```python
from build123d import *

# Parameters (mm, degrees)
SKETCH1_W                     = 100
SKETCH1_H                     = 400
BOSS_EXTRUDE1_DEPTH           = 3.175
M4_CLEARANCE_HOLE2_D          = 4.5
SKETCH7_W                     = 400
SKETCH7_H                     = 3.175
BOSS_EXTRUDE2_DEPTH           = 20
M4_CLEARANCE_HOLE1_D          = 4.5
SKETCH13_W                    = 17.5
SKETCH13_H                    = 265
SKETCH13_W_2                  = 58
SKETCH13_H_2                  = 69.5
SKETCH13_W_3                  = 4.5
SKETCH13_H_3                  = 66
SKETCH13_H_4                  = 10
SKETCH13_H_5                  = 29.5
SKETCH13_H_6                  = 75
CUT_EXTRUDE1_DEPTH            = 3.175
FILLET1_R                     = 10
SKETCH14_W                    = 120
SKETCH14_H                    = 250.5
CUT_EXTRUDE2_DEPTH            = 3.175
M4_CLEARANCE_HOLE3_AT_2_COUNT = 2
M4_CLEARANCE_HOLE3_AT_2_PITCH = 26.666666667


with BuildPart() as part:
    # Sketch1 → Boss-Extrude1 (new body)
    with BuildSketch(Plane(origin=(0, 0, 0), x_dir=(1, 0, 0), z_dir=(0, 1, 0))):
        Rectangle(SKETCH1_W, SKETCH1_H)
    extrude(amount=BOSS_EXTRUDE1_DEPTH)

    # M4 Clearance Hole2 (through all)
    with Locations(Plane(origin=(0, 3.175, 0), x_dir=(1, 0, 0), z_dir=(0, 1, 0))):
        with Locations((-40, 190), (40, 190), (40, -190), (-40, -190), (-40, 95), (40, 95)):
            Hole(M4_CLEARANCE_HOLE2_D / 2)

    # Sketch7 → Boss-Extrude2 (add)
    with BuildSketch(Plane(origin=(50, 0, 0), x_dir=(0, 0, -1), z_dir=(1, 0, 0))):
        with Locations((0, 1.5875)):
            Rectangle(SKETCH7_W, SKETCH7_H)
    extrude(amount=BOSS_EXTRUDE2_DEPTH)

    # M4 Clearance Hole1 (through all)
    with Locations(Plane(origin=(0, 3.175, 0), x_dir=(1, 0, 0), z_dir=(0, 1, 0))):
        with Locations((55.5, -140.5), (55.5, -110.5), (-22.5, -110.5), (-22.5, -140.5), (-22.5, -24.5), (-22.5, 5.5), (55.5, 5.5), (55.5, -24.5)):
            Hole(M4_CLEARANCE_HOLE1_D / 2)

    # Sketch13 → Cut-Extrude1 (cut)
    with BuildSketch(Plane(origin=(0, 3.175, 0), x_dir=(1, 0, 0), z_dir=(0, 1, 0))):
        with Locations((-41.25, -47.5)):
            Rectangle(SKETCH13_W, SKETCH13_H)
        with Locations((16.5, 50.25)):
            Rectangle(SKETCH13_W_2, SKETCH13_H_2)
        with Locations((67.75, -47.5)):
            Rectangle(SKETCH13_W_3, SKETCH13_H)
        with Locations((16.5, -67.5)):
            Rectangle(SKETCH13_W_2, SKETCH13_H_3)
        with Locations((16.5, -125.5)):
            Rectangle(SKETCH13_W_2, SKETCH13_H_4)
        with Locations((16.5, -165.25)):
            Rectangle(SKETCH13_W_2, SKETCH13_H_5)
        with Locations((-41.25, 142.5)):
            Rectangle(SKETCH13_W, SKETCH13_H_6)
        with Locations((16.5, 142.5)):
            Rectangle(SKETCH13_W_2, SKETCH13_H_6)
        with Locations((67.75, 142.5)):
            Rectangle(SKETCH13_W_3, SKETCH13_H_6)
        with Locations((16.5, -9.5)):
            Rectangle(SKETCH13_W_2, SKETCH13_H_4)
    extrude(amount=-CUT_EXTRUDE1_DEPTH, mode=Mode.SUBTRACT)

    # Fillet1
    # the kernel refuses this fillet: 10 mm, written as the material it takes off along each edge
    with BuildSketch(Plane(origin=(70, 24.054116361, -180), x_dir=(0, 0, -1), z_dir=(0, -1, 0)), Plane(origin=(70, 24.054116361, -85), x_dir=(0, 0, -1), z_dir=(0, -1, 0))) as fillet1_piece_1:
        with BuildLine():
            CenterArc((8.351646544, -10), FILLET1_R, 90, 56.632987031)
            Line((0, -4.5), (-0.167032931, -4.39))
            ThreePointArc((-0.167032931, -4.39), (-0.2, -2.25), (-0.2, 0))
            Line((-0.2, 0), (0, 0.2))
            Line((0, 0.2), (8.351646544, 0.2))
            Line((8.351646544, 0.2), (8.351646544, 0))
        make_face()
    extrude(amount=44.933232721, mode=Mode.SUBTRACT)
    with BuildSketch(Plane(origin=(70, -25, -200), x_dir=(-1, 0, 0), z_dir=(0, 1, 0)), Plane(origin=(-50, -25, -200), x_dir=(0, 0, 1), z_dir=(0, 1, 0)), Plane(origin=(70, 28.175, 200), x_dir=(-1, 0, 0), z_dir=(0, -1, 0)), Plane(origin=(-50, -25, 200), x_dir=(1, 0, 0), z_dir=(0, 1, 0))) as fillet1_piece_2:
        with BuildLine():
            CenterArc((FILLET1_R, FILLET1_R), FILLET1_R, 180, 90)
            Line((0, FILLET1_R), (-FILLET1_R * 0.02, FILLET1_R))
            Line((-FILLET1_R * 0.02, FILLET1_R), (-FILLET1_R * 0.02, -FILLET1_R * 0.02))
            Line((-FILLET1_R * 0.02, -FILLET1_R * 0.02), (FILLET1_R, -FILLET1_R * 0.02))
            Line((FILLET1_R, -FILLET1_R * 0.02), (FILLET1_R, 0))
        make_face()
    extrude(amount=53.175, mode=Mode.SUBTRACT)
    with BuildSketch(Plane(origin=(-50, 28.175, -180), x_dir=(1, 0, 0), z_dir=(0, -1, 0)), Plane(origin=(-50, 28.175, -85), x_dir=(1, 0, 0), z_dir=(0, -1, 0)), Plane(origin=(-50, 28.175, -105), x_dir=(0, 0, 1), z_dir=(0, -1, 0)), Plane(origin=(-50, 28.175, 180), x_dir=(0, 0, 1), z_dir=(0, -1, 0))) as fillet1_piece_3:
        with BuildLine():
            CenterArc((FILLET1_R, -FILLET1_R), FILLET1_R, 90, 90)
            Line((0, -FILLET1_R), (-FILLET1_R * 0.02, -FILLET1_R))
            Line((-FILLET1_R * 0.02, -FILLET1_R), (-FILLET1_R * 0.02, FILLET1_R * 0.02))
            Line((-FILLET1_R * 0.02, FILLET1_R * 0.02), (FILLET1_R, FILLET1_R * 0.02))
            Line((FILLET1_R, FILLET1_R * 0.02), (FILLET1_R, 0))
        make_face()
    extrude(amount=53.175, mode=Mode.SUBTRACT)
    with BuildSketch(Plane(origin=(70, 24.054116361, -105), x_dir=(-1.0, 0, 1.5347723092402606e-12), z_dir=(0, -1, 0))) as fillet1_piece_4:
        with BuildLine():
            CenterArc((10, -8.351646544), FILLET1_R, 123.367012969, 56.632987031)
            Line((0, -8.351646544), (-0.2, -8.351646544))
            Line((-0.2, -8.351646544), (-0.2, 0))
            Line((-0.2, 0), (0, 0.2))
            ThreePointArc((0, 0.2), (2.25, 0.2), (4.39, 0.167032931))
            Line((4.39, 0.167032931), (4.5, 0))
        make_face()
    extrude(amount=44.933232721, mode=Mode.SUBTRACT)
    with BuildSketch(Plane(origin=(70, 24.054116361, 180), x_dir=(0, 0, 1), z_dir=(0, -1, 0))) as fillet1_piece_5:
        with BuildLine():
            CenterArc((8.351646544, 10), FILLET1_R, 213.367012969, 56.632987031)
            Line((0, 4.5), (-0.167032931, 4.39))
            ThreePointArc((-0.167032931, 4.39), (-0.2, 2.25), (-0.2, 0))
            Line((-0.2, 0), (0, -0.2))
            Line((0, -0.2), (8.351646544, -0.2))
            Line((8.351646544, -0.2), (8.351646544, 0))
        make_face()
    extrude(amount=44.933232721, mode=Mode.SUBTRACT)

    # Sketch14 → Cut-Extrude2 (cut)
    with BuildSketch(Plane(origin=(0, 3.175, 0), x_dir=(1, 0, 0), z_dir=(0, 1, 0))):
        with Locations((10, 74.75)):
            Rectangle(SKETCH14_W, SKETCH14_H)
    extrude(amount=-CUT_EXTRUDE2_DEPTH, mode=Mode.SUBTRACT)

    # Sketch16 → M4 Clearance Hole3 (revolve, cut)
    with BuildSketch(Plane(origin=(13.333333333, 0, 190), x_dir=(0, 0, -1), z_dir=(1, 0, 0))):
        Polygon((0, 0), (0, 3.175), (2.275, 3.175), (2.25, 3.15), (2.25, 0.025), (2.275, 0), align=None)
    m4_clearance_hole3 = revolve(axis=Axis((13.333333333, -6.35, 190), (0, 1, 0)), mode=Mode.SUBTRACT)

    # M4 Clearance Hole3 at 2: M4 Clearance Hole3 ×2
    with Locations(*[(-i * M4_CLEARANCE_HOLE3_AT_2_PITCH, 0, 0) for i in range(1, M4_CLEARANCE_HOLE3_AT_2_COUNT)]):
        add(m4_clearance_hole3, mode=Mode.SUBTRACT)


solid = part.part
```
Geometry check sheet. Reference: the model listing, model coordinates, mm. A direction names the side the tool comes from. Give positions to 0.01 mm unless a question says otherwise; leave off trailing zeros. Order: outer loops, then holes, each group sorted by start corner. A loop starts at its lowest first (then second) coordinate and runs counter-clockwise, first axis right, second up. Notation, with made-up numbers: (61.5, 59.5) -> (106.5, 59.5) arc R22 cw to (106.5, 85.5) -> close; hole circle Ø4 at (-24, -12). An arc over 180 degrees is marked (long way). Write each question's results on one line, items separated by ' | '. Start each with the question number.
(1) Gauge pin test, flat ends, axial feed: P1, Ø1.5, axis at y = 2.5, z = 129, coming from the -X side; P2, Ø1.6, axis at x = -36.5, y = 1, coming from the -Z side; P3, Ø1.6, axis at y = 1.5, z = 101, coming from the +X side. Record the tip position at first contact, or that the pin passes through.
(2) Sectioned sample at D-D (x = 40). Enter the section's corners in (y, z) (3 decimals), plus the area to 3 significant figures.
(3) Sectioned sample at B-B (z = 140.5). Enter the section's corners in (x, y) (3 decimals).
(4) Scan lines: line 1 (X direction, y = 1.1, z = 190); line 2 (Z direction, x = 40, y = 1.7); line 3 (Z direction, x = 25, y = 1.95). Record each from-to range of solid material in increasing order.
(5) Sectioned sample at A-A (x = 8.5). Enter the section's corners in (y, z) (3 decimals), plus the area to 4 significant figures.
(6) Sectioned sample at C-C (z = 159.5). Enter the section's corners in (x, y) (3 decimals).
(7) Access from +Z, -Z, +X, -X, +Y, -Y to the whole of each face (thin tool, end or side, straight path). Record for faces 1 (the face through (9, 0, 143)), 2 (the face through (-36, 2, 180)), 3 (the face through (-12.5, 2, 165)).
(8) Mould release check, pull along X, two halves, no side actions. Record for faces 4 (the face through (67.15, 1.61, 196.99)), 5 (the face through (-12.5, 2, 126)), 6 (the face through (9, 2, 200)): pulls with the +X half, pulls with the -X half, needs draft (parallel to the pull), parting line crosses it, or undercut.
Answer below:
1) P1: x = -32.5 | P2: z = 180 | P3: x = 65.5
2) outline: (0, 100.5) -> (3.175, 100.5) -> (3.175, 120.5) -> (0, 120.5) -> close; (0, 130.5) -> (3.175, 130.5) -> (3.175, 150.5) -> (0, 150.5) -> close; (0, 180) -> (3.175, 180) -> (3.175, 187.75) -> (0, 187.75) -> close; (0, 192.25) -> (3.175, 192.25) -> (3.175, 200) -> (0, 200) -> close | area: 176 mm2
3) outline: (-32.5, 0) -> (-24.75, 0) -> (-24.75, 3.175) -> (-32.5, 3.175) -> close; (-20.25, 0) -> (53.25, 0) -> (53.25, 3.175) -> (-20.25, 3.175) -> close; (57.75, 0) -> (65.5, 0) -> (65.5, 3.175) -> (57.75, 3.175) -> close
4) line 1: -50 to -42.25, -37.75 to -15.58, -11.08 to 11.08, 15.58 to 37.75, 42.25 to 70 | line 2: 100.5 to 120.5, 130.5 to 150.5, 180 to 187.75, 192.25 to 200 | line 3: 100.5 to 120.5, 130.5 to 150.5, 180 to 200
5) outline: (0, 100.5) -> (3.175, 100.5) -> (3.175, 120.5) -> (0, 120.5) -> close; (0, 130.5) -> (3.175, 130.5) -> (3.175, 150.5) -> (0, 150.5) -> close; (0, 180) -> (3.175, 180) -> (3.175, 200) -> (0, 200) -> close | area: 190.5 mm2
6) outline: (-32.5, 0) -> (-12.5, 0) -> (-12.5, 3.175) -> (-32.5, 3.175) -> close; (45.5, 0) -> (65.5, 0) -> (65.5, 3.175) -> (45.5, 3.175) -> close
7) face 1: +Z, -Z, +X, -X, -Y | face 2: -Z, -X, +Y, -Y | face 3: +Y, -Y
8) face 4: pulls with the +X half | face 5: undercut | face 6: needs draft
